Design review of the part built by this model. Coordinates are the model's own, in mm. Face numbers are marked on the shaded views. A direction names the side the tool comes from. Coordinates: 2 decimals unless noted, no trailing zeros. Loops run counter-clockwise (first coordinate to the right, second up) from the corner with the lowest first, then second, coordinate; pieces in that order, holes last. Notation, with made-up numbers: (45, 15.5) -> (66, 15.5) arc R18 cw to (66, 43.5) -> close; hole circle Ø5 at (76, 55.25). An arc over 180 degrees is marked (long way). Use a Markdown table: item, result. Add a question column.
Q1. Clearance check with flat-ended pins moving along their axes: pin 1 Ø0.8 at (x, z) = (49.5, 28.5) entering from -Y; pin 2 Ø3.5 at (x, y) = (4.5, 9) entering from +Z; pin 3 Ø12 at (x, z) = (30.5, 19) entering from -Y; pin 4 Ø1.1 at (x, z) = (49.5, 28) entering from +Y. State where each tip first meets the part, or that it passes through.
Q2. For the marked faces 1 and 2, list the 3-axis set-ups (+Z, -Z, +X, -X, +Y, -Y) from which the entire face can be reached by the end or side of a thin tool; tool diameter is ignored.
Q3. Draft analysis for pull direction X (two halves, no side actions). For the marked faces 3, 4, 5 and 6, state which applies: pulls with the +X half, pulls with the -X half, needs draft (parallel to the pull), parting line crosses it, or undercut.
Q4. Take a section at A-A on z = 28.5. Write out the cut boundary in (x, y).
Q5. For probe 1 along Z at (x, y) = (42, 40); probe 2 along Z at (x, y) = (22.5, 4); probe 3 along X at (y, z) = (6, 17), list the stretches that pass through material, from the lowest coordinate up.
Q6. Take a section at B-B on y = 40. Write out the cut boundary in (x, z), plus the area to 3 significant figures.
from build123d import *

# Parameters (mm, degrees)
SKETCH1_W                = 50
SKETCH1_H                = 50
BOSS_EXTRUDE1_DEPTH      = 25
CHAMFER1_SIZE            = 1.5
BOSS_EXTRUDE2_DEPTH      = 7
BOSS_EXTRUDE2_DEPTH_BACK = 10
SKETCH5_W                = 1
SKETCH5_H                = 7
SKETCH6_W                = 1.8
SKETCH6_H                = 1.8
CUT_EXTRUDE1_DEPTH       = 7


with BuildPart() as part:
    # Sketch1 → Boss-Extrude1 (new body)
    with BuildSketch(Plane.XY):
        with Locations((25, 25)):
            Rectangle(SKETCH1_W, SKETCH1_H)
    extrude(amount=BOSS_EXTRUDE1_DEPTH)

    # Cut-Sweep1: sweep along a path in Sketch4
    with BuildLine(Plane.XY.offset(25)) as cut_sweep1_path:
        Line((25, 0), (25, 3))
        ThreePointArc((25, 3), (18.556349186, 18.556349186), (3, 25))
        Line((3, 25), (0, 25))
    # Sketch3 → Cut-Sweep1 (sweep, cut)
    with BuildSketch(Plane.XZ):
        Polygon((36, 29.556349186), (29.556349186, 36), (20.443650814, 36), (14, 29.556349186), (14, 20.443650814), (20.443650814, 14), (29.556349186, 14), (36, 20.443650814), align=None)
    sweep(path=cut_sweep1_path.line, mode=Mode.SUBTRACT)

    # Chamfer1
    chamfer1_edges = [part.edges().sort_by_distance(p)[0] for p in [
        (50, 25, 25),
        (25, 50, 25),
        (0, 7, 25),
        (43, 0, 25),
        (14, 1.5, 25),
        (10.778174593, 10.778174593, 25),
        (1.5, 14, 25),
        (36, 1.5, 25),
        (26.334523779, 26.334523779, 25),
        (1.5, 36, 25),
        (0, 14, 22.721825407),
        (0, 36, 22.721825407),
        (36, 0, 22.721825407),
        (14, 0, 22.721825407),
        (17.221825407, 0, 17.221825407),
        (32.778174593, 0, 17.221825407),
        (0, 32.778174593, 17.221825407),
        (0, 17.221825407, 17.221825407),
        (0, 43, 25),
        (25, 50, 0),
        (50, 25, 0),
        (25, 0, 0),
        (0, 25, 0),
        (7, 0, 25),
        (0, 50, 12.5),
        (50, 50, 12.5),
        (50, 0, 12.5),
        (0, 0, 12.5),
    ]]
    chamfer(chamfer1_edges, length=CHAMFER1_SIZE)

    # Sketch5 → Boss-Extrude2 (add, two sides: drawn at the far end of the back side and taken through both)
    with BuildSketch(Plane.XY.offset(25).offset(-BOSS_EXTRUDE2_DEPTH_BACK)):
        with Locations((49.5, 25)):
            Rectangle(SKETCH5_W, SKETCH5_H)
    extrude(amount=BOSS_EXTRUDE2_DEPTH + BOSS_EXTRUDE2_DEPTH_BACK)

    # Sketch6 → Cut-Extrude1 (cut)
    with BuildSketch(Plane(origin=(50, 0, 0), x_dir=(0, 0, -1), z_dir=(1, 0, 0))):
        with Locations((-28.6, 25)):
            Rectangle(SKETCH6_W, SKETCH6_H)
    extrude(amount=-CUT_EXTRUDE1_DEPTH, mode=Mode.SUBTRACT)


solid = part.part
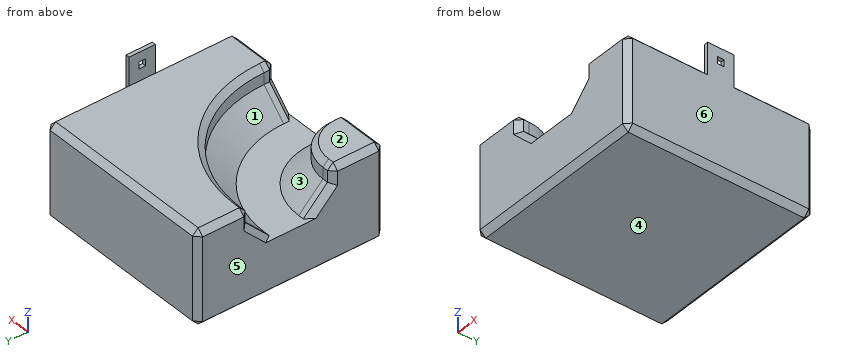
Answer list:
| question | item | result |
|---|---|---|
| 1 | pin 1 | y = 21.5 |
| 1 | pin 2 | z = 25 |
| 1 | pin 3 | y = 0 |
| 1 | pin 4 | y = 28.5 |
| 2 | face 1 | +Z |
| 2 | face 2 | +Z, +X, -X, +Y, -Y |
| 3 | face 3 | undercut |
| 3 | face 4 | needs draft |
| 3 | face 5 | pulls with the -X half |
| 3 | face 6 | pulls with the +X half |
| 4 | outline | (49, 21.5) -> (50, 21.5) -> (50, 24.1) -> (49, 24.1) -> close; (49, 25.9) -> (50, 25.9) -> (50, 28.5) -> (49, 28.5) -> close |
| 5 | probe 1 | 0 to 25 |
| 5 | probe 2 | 0 to 14 |
| 5 | probe 3 | 0 to 17.13, 32.4 to 50 |
| 6 | outline | (0, 1.5) -> (1.5, 0) -> (48.5, 0) -> (50, 1.5) -> (50, 23.5) -> (48.5, 25) -> (1.5, 25) -> (0, 23.5) -> close |
| 6 | area | 1,250 mm² |
